from build123d import *

# Parameters (mm, degrees)
SKETCH1_W           = 5.46
SKETCH1_H           = 4.09
BOSS_EXTRUDE1_DEPTH = 1.105
BOSS_EXTRUDE2_START = -7.5
SKETCH2_R           = 0.4
BOSS_EXTRUDE2_DEPTH = 10


with BuildPart() as part:
    # Sketch1 → Boss-Extrude1 (new, symmetric)
    with BuildSketch(Plane.XY):
        Rectangle(SKETCH1_W, SKETCH1_H)
    extrude(amount=BOSS_EXTRUDE1_DEPTH, both=True)

    # Sketch2 → Boss-Extrude2 (add)
    with BuildSketch(Plane(origin=(0, 2.045, 0), x_dir=(1, 0, 0), z_dir=(0, 1, 0)).offset(BOSS_EXTRUDE2_START)):
        with Locations(Location((-1.905, 0, 0), (0, 0, 270))):
            Circle(SKETCH2_R)
        with Locations(Location((-0.635, 0, 0), (0, 0, 270))):
            Circle(SKETCH2_R)
        with Locations(Location((0.635, 0, 0), (0, 0, 270))):
            Circle(SKETCH2_R)
        with Locations(Location((1.905, 0, 0), (0, 0, 270))):
            Circle(SKETCH2_R)
    extrude(amount=BOSS_EXTRUDE2_DEPTH)


solid = part.part
Read the model definition and answer for the solid it produces. Units are mm, in the model's axes. A direction names the side the tool comes from. Round coordinates to 2 decimals unless told otherwise and drop trailing zeros. Write each loop counter-clockwise with the first axis right and the second up, starting at its lowest first coordinate (ties: lowest second). Pieces come first, ordered by that corner, then holes. Notation, with made-up numbers: (16.25, 14.25) - (71.25, 14.25) arc R20 ccw to (71.25, 32.25) - close; hole circle Ø9 at (61.25, 27.25). An arc over 180 degrees is marked (long way). Use a Markdown table: item, result.
(1) The part is cut by section C-C (y = -4.5). Write down the section's boundary in (x, z) (3 decimals).
Reported:
| item | result |
|---|---|
| outline | circle Ø0.8 at (-1.905, 0); circle Ø0.8 at (-0.635, 0); circle Ø0.8 at (0.635, 0); circle Ø0.8 at (1.905, 0) |
(2) The part is cut by section B-B (z = -0.9). Write down the section's boundary in (x, y) (3 decimals), then the cut area to 3 significant figures.
Reported:
| item | result |
|---|---|
| outline | (-2.73, -2.045) - (2.73, -2.045) - (2.73, 2.045) - (-2.73, 2.045) - close |
| area | 22.3 mm2 |
(3) The mould has two halves that part along X. Classify faces 1 (the flat face through (2.73, 0, 0)), 2 (the flat face through (-2.73, 0, 0)), 3 (the cylindrical face through (-2.26, 3.28, 0.18)): released by +X, released by -X, zero draft, split by the parting line, or undercut.
Reported:
| item | result |
|---|---|
| face 1 | released by +X |
| face 2 | released by -X |
| face 3 | undercut |
(4) Straight lines are drawn through the part: line 1 along X through (y, z) = (-4.5, -0.2); line 2 along X through (y, z) = (-5, -0.3); line 3 along Y through (x, z) = (1.95, 0.6) (3 decimals). For each, find the intervals that lie inside material, in ascending order. Write a range as [from, to].
Reported:
| item | result |
|---|---|
| line 1 | [-2.25, -1.56], [-0.98, -0.29], [0.29, 0.98], [1.56, 2.25] |
| line 2 | [-2.17, -1.64], [-0.9, -0.37], [0.37, 0.9], [1.64, 2.17] |
| line 3 | [-2.045, 2.045] |
(5) Which of the six approach directions +Z, -Z, +X, -X, +Y, -Y give full straight-line access (tool end or side, diameter ignored) to faces 4 (the cylindrical face through (-2.26, -3.77, 0.18)), 5 (the flat face through (0, 0, -1.105)), 6 (the flat face through (0, 2.045, 0))?
Reported:
| item | result |
|---|---|
| face 4 | -Y |
| face 5 | -Z, +X, -X, +Y, -Y |
| face 6 | +Y |
(6) This flat-tipped pin is pushed along its axis until it touches: pin 1 Ø2 at (x, y) = (1.5, -3.5) entering from +Z. Where does it stop, or does it pass through?
Reported:
| item | result |
|---|---|
| pin 1 | z = 0.4 |
(7) The part is cut by section A-A (x = -1.75). Write down the section's boundary in (y, z) (3 decimals).
Reported:
| item | result |
|---|---|
| outline | (-5.455, -0.369) - (-2.045, -0.369) - (-2.045, -1.105) - (2.045, -1.105) - (2.045, -0.369) - (4.545, -0.369) - (4.545, 0.369) - (2.045, 0.369) - (2.045, 1.105) - (-2.045, 1.105) - (-2.045, 0.369) - (-5.455, 0.369) - close |
(8) The part is cut by section D-D (x = 2.15). Write down the section's boundary in (y, z) (3 decimals), then the cut area to 3 significant figures.
Reported:
| item | result |
|---|---|
| outline | (-5.455, -0.316) - (-2.045, -0.316) - (-2.045, -1.105) - (2.045, -1.105) - (2.045, -0.316) - (4.545, -0.316) - (4.545, 0.316) - (2.045, 0.316) - (2.045, 1.105) - (-2.045, 1.105) - (-2.045, 0.316) - (-5.455, 0.316) - close |
| area | 12.8 mm2 |
